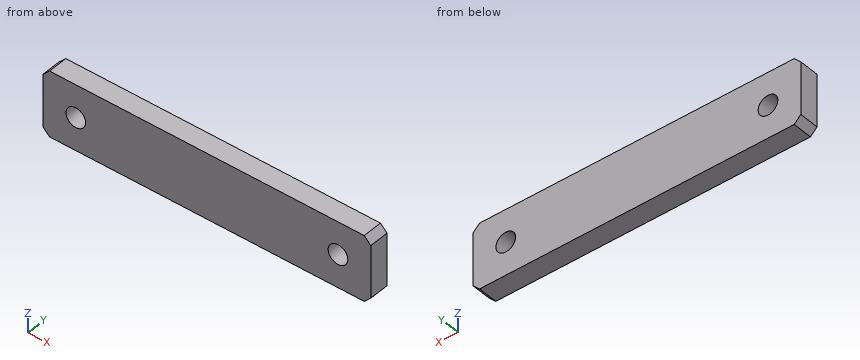
from build123d import *

# Parameters (mm, degrees)
F0_W     = 50
F0_H     = 10
F1_DEPTH = 3
F2_R     = 1.5
F3_DEPTH = 5
F4_SIZE  = 1


with BuildPart() as f1:
    # F0 (on Front) → F1 (new body)
    with BuildSketch(Plane.XZ):
        with Locations((-25, 5)):
            Rectangle(F0_W, F0_H)
    extrude(amount=F1_DEPTH)

    # F2 (on face) → F3 (cut)
    with BuildSketch(Plane.XZ.offset(3)):
        with Locations((-45, 5)):
            Circle(F2_R)
        with Locations((-5, 5.036021)):
            Circle(F2_R)
    extrude(amount=-F3_DEPTH, mode=Mode.SUBTRACT)

    # F4
    f4_edges = [f1.edges().sort_by_distance(p)[0] for p in [
        (0, -1.5, 10),
        (0, -1.5, 0),
        (-50, -1.5, 10),
        (-50, -1.5, 0),
    ]]
    chamfer(f4_edges, length=F4_SIZE)


solid = f1.part
Check sheet for the modelled part. Datum: model origin and axes. Units: mm. Give positions to 0.01 mm unless a question says otherwise; leave off trailing zeros. Loops run counter-clockwise (first coordinate to the right, second up) from the corner with the lowest first, then second, coordinate; pieces in that order, holes last. Notation, with made-up numbers: M 27.25,76 L 82.25,76 A13 cw 82.25,89 Z; hole C -32.75,66.5 d7. An arc over 180 degrees is marked long. Return JSON: item names as keys, results as strings. Group by question number.
1. Thickness scan on L1, parallel to X at y = -1.9, z = 6; L2, parallel to X at y = -2.7, z = 5.25; L3, parallel to Z at x = -45, y = -2.2. Record the ranges inside material, lowest first.
2. Cross-section at B-B on y = -1.5. Record the boundary of the cut face in (x, z), plus the area to 3 significant figures.
3. Go/stop test with a flat-tipped pin: pin 1 (2.5 mm diameter, centred on x = -5, z = 5.04, fed in from -Y) (3 decimals). Record where the tip stops, or that it passes through.
4. Cross-section at A-A on x = -5. Record the boundary of the cut face in (y, z), plus the area to 3 significant figures.
Return value:
{
 "1": {"L1": "-50 to -46.12, -43.88 to -6.15, -3.85 to 0", "L2": "-50 to -46.48, -43.52 to -6.48, -3.52 to 0", "L3": "0 to 3.5, 6.5 to 10"},
 "2": {"outline": "M -50,1 L -49,0 L -1,0 L 0,1 L 0,9 L -1,10 L -49,10 L -50,9 Z; hole C -45,5 d3; hole C -5,5.04 d3", "area": "484 mm^2"},
 "3": {"pin 1": "through"},
 "4": {"outline": "M -3,0 L 0,0 L 0,3.54 L -3,3.54 Z; M -3,6.54 L 0,6.54 L 0,10 L -3,10 Z", "area": "21.0 mm^2"}
}
